Geometry check sheet. Reference: the model listing, model coordinates, mm. Give positions to 0.01 mm unless a question says otherwise; leave off trailing zeros. Loops run counter-clockwise (first coordinate to the right, second up) from the corner with the lowest first, then second, coordinate; pieces in that order, holes last. Notation, with made-up numbers: (8.25, 53.5) - (38.25, 53.5) arc R26 ccw to (38.25, 90.5) - close; hole circle Ø3 at (48, -7.5). An arc over 180 degrees is marked (long way). Use a Markdown table: item, result. Add a question column.
1. Draft check along Z on faces 1 (the flat face through (34, 0, -7)), 2 (the cylindrical face through (63, 0, 0)), 3 (the cylindrical face through (75, 0, 0)). Enter one of: pulls with the +Z half, pulls with the -Z half, needs draft (parallel to the pull), parting line crosses it, or undercut.
2. Cross-section at B-B on y = 0.2. Enter the section's corners in (x, z).
3. Material ranges on L1, parallel to Z at x = 0, y = 0.55; L2, parallel to X at y = 1.3, z = -0.25; L3, parallel to X at y = -1.3, z = 3.25, recorded low to high.
4. Cross-section at C-C on z = -4. Enter the section's corners in (x, y).
5. Cross-section at A-A on z = 0. Enter the section's corners in (x, y).
6. Depth check by flat-ended pin: P1, Ø1, axis at y = 0, z = 1, coming from the -X side. Enter the tip coordinate at first touch or a pass-through.
Solid Edge part; units mm, degrees
sketch "Sketch1" plane through (0, 0, 0) normal (0, -1, 0) x (1, 0, 0)
  circle A0 centre (0, 0) radius 5
  line L0 (0, 7) -> (68.0003, 7)
  line L1 (0, -7) -> (68.0003, -7)
  arc A1 (0, -7) -> (0, 7) centre (0, 0) cw
  arc A2 (68.0003, 7) -> (68.0003, -7) centre (68.0003, 0) cw
  circle A3 centre (68.0003, 0) radius 5
extrude "Protrusion1" add sketch "Sketch1" along normal mid plane 3
properties part number "1976-1500-004" material "Aluminio, 7075-T6"
Values found:
| question | item | result |
|---|---|---|
| 1 | face 1 | pulls with the -Z half |
| 1 | face 2 | undercut |
| 1 | face 3 | parting line crosses it |
| 2 | outline | (0, -7) - (68, -7) arc R7 ccw to (68, 7) - (0, 7) arc R7 ccw to start; hole circle Ø10 at (0, 0); hole circle Ø10 at (68, 0) |
| 3 | L1 | z = -7 to -5, 5 to 7 |
| 3 | L2 | x = -7 to -4.99, 4.99 to 63.01, 72.99 to 75 |
| 3 | L3 | x = -6.2 to -3.8, 3.8 to 64.2, 71.8 to 74.2 |
| 4 | outline | (-5.74, -1.5) - (-3, -1.5) - (-3, 1.5) - (-5.74, 1.5) - close; (3, -1.5) - (65, -1.5) - (65, 1.5) - (3, 1.5) - close; (71, -1.5) - (73.74, -1.5) - (73.74, 1.5) - (71, 1.5) - close |
| 5 | outline | (-7, -1.5) - (-5, -1.5) - (-5, 1.5) - (-7, 1.5) - close; (5, -1.5) - (63, -1.5) - (63, 1.5) - (5, 1.5) - close; (73, -1.5) - (75, -1.5) - (75, 1.5) - (73, 1.5) - close |
| 6 | P1 | stops at x = -6.98 |
